Here's the drawing with two shaded views (mm, measured from the low corner). I have some questions. A direction names the side the tool comes from. Coordinates: 2 decimals unless noted, no trailing zeros. Loops run counter-clockwise (first coordinate to the right, second up) from the corner with the lowest first, then second, coordinate; pieces in that order, holes last.
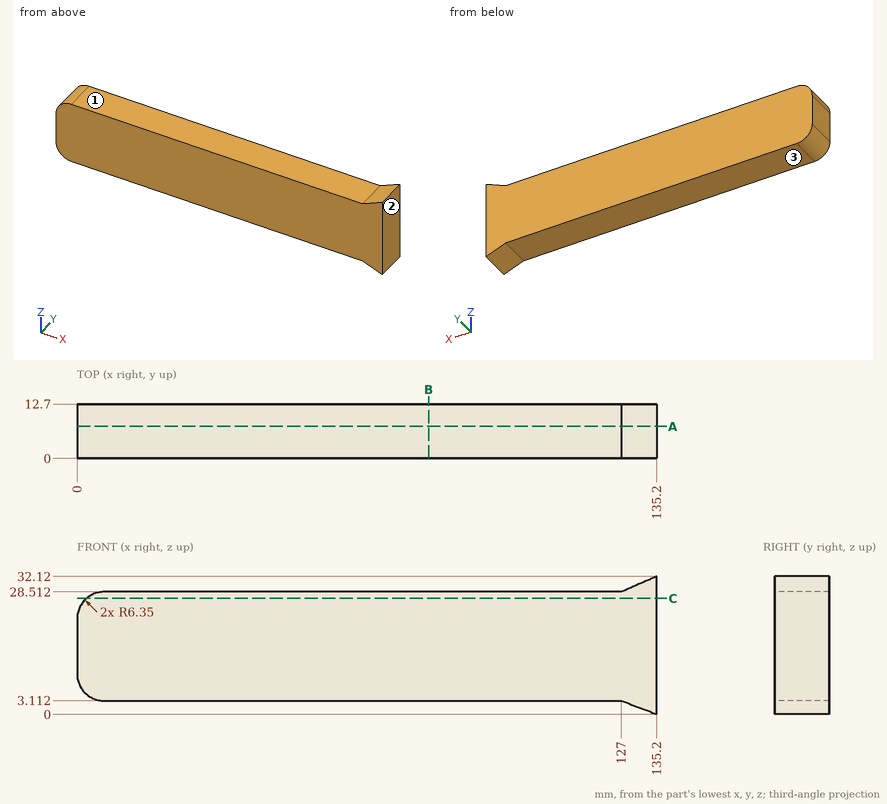
(1) I'm going to push a flat-ended pin straight in: pin 1 (6.5 mm diameter, centred on x = 77, y = 4.5, fed in from -Z). Where does the tip first touch, or does it pass through?
Check values:
pin 1: stops at z = 3.11
(2) I want a section at A-A on y = 7.5. Write out the boundary of the cut face in (x, z).
Check values:
outline: (0, 9.46) arc R6.35 ccw to (6.35, 3.11) - (127, 3.11) - (135.2, 0) - (135.2, 32.12) - (127, 28.51) - (6.35, 28.51) arc R6.35 ccw to (0, 22.16) - close
(3) Which directions (+Z, -Z, +X, -X, +Y, -Y) give clear straight access to the entire face, cutting with the end or side of a thin tool? Please do the marked faces 1, 2 and 3.
Check values:
face 1: +Z, -X, +Y, -Y
face 2: +Z, -Z, +X, +Y, -Y
face 3: -Z, -X, +Y, -Y
(4) I want a section at B-B on x = 82. Write out the boundary of the cut face in (y, z).
Check values:
outline: (0, 3.11) - (12.7, 3.11) - (12.7, 28.51) - (0, 28.51) - close
(5) If I drill on probe 1 along Z at (x, y) = (50.5, 2.5); probe 2 along X at (y, z) = (6.5, 29.5) (1 decimal); probe 3 along X at (y, z) = (6, 27.5), over which ranges is the centre line in solid material (lowest first)?
Check values:
probe 1: z = 3.11 to 28.51
probe 2: x = 129.2 to 135.2
probe 3: x = 2.91 to 135.2
(6) I want a section at C-C on z = 27. Write out the boundary of the cut face in (x, y).
Check values:
outline: (2.24, 0) - (135.2, 0) - (135.2, 12.7) - (2.24, 12.7) - close
